Check sheet for the modelled part. Datum: model origin and axes. Units: mm. Face numbers are marked on the shaded views. Coordinates: 2 decimals unless noted, no trailing zeros. Loops run counter-clockwise (first coordinate to the right, second up) from the corner with the lowest first, then second, coordinate; pieces in that order, holes last. Notation, with made-up numbers: (1.25, -15) - (47.25, -15) arc R23 ccw to (47.25, -3) - close; hole circle Ø8 at (50, -14.5). An arc over 180 degrees is marked (long way). Use a Markdown table: item, result. Add a question column.
1) Thickness scan on line 1 (Z direction, x = -3, y = 9.5); line 2 (X direction, y = 9.5, z = -21.5); line 3 (Z direction, x = 2, y = 3.25). Record the ranges inside material, lowest first.
2) Go/stop test with flat-tipped pins: P1, Ø4.5, axis at x = 14, z = -68.5, coming from the +Y side; P2, Ø1.5, axis at y = 5, z = -24, coming from the +X side; P3, Ø1, axis at x = 10.5, y = 12, coming from the -Z side. Record where each tip stops, or that it passes through.
3) Draft check along Y on the marked faces 1, 2, 3 and 4. Enter one of: pulls with the +Y half, pulls with the -Y half, needs draft (parallel to the pull), parting line crosses it, or undercut.
4) Sectioned sample at B-B, the plane x = -0.75. Enter the section's corners in (y, z), then the cut area to 3 significant figures.
5) Sectioned sample at A-A, the plane y = 7.5. Enter the section's corners in (x, z).
6) Sectioned sample at C-C, the plane z = -52.5. Enter the section's corners in (x, y), then the cut area to 3 significant figures.
from build123d import *

# Parameters (mm, degrees)
SKETCH1_W           = 85.2
SKETCH1_H           = 18
SKETCH1_W_2         = 10
SKETCH1_H_2         = 12
BOSS_EXTRUDE1_DEPTH = 9
SKETCH2_W           = 5
SKETCH2_H           = 12
BOSS_EXTRUDE2_DEPTH = 6
FILLET1_R           = 2
FILLET2_R           = 1
FILLET3_R           = 4


with BuildPart() as part:
    # Sketch1 → Boss-Extrude1 (new, symmetric)
    with BuildSketch(Plane(origin=(0, 0, 0), x_dir=(0, 0, -1), z_dir=(1, 0, 0))):
        with Locations((42.6, 9)):
            Rectangle(SKETCH1_W, SKETCH1_H)
        with Locations((76.2, 9)):
            Rectangle(SKETCH1_W_2, SKETCH1_H_2, mode=Mode.SUBTRACT)
    extrude(amount=BOSS_EXTRUDE1_DEPTH, both=True)

    # Sketch2 → Boss-Extrude2 (add)
    with BuildSketch(Plane(origin=(9, 0, 0), x_dir=(0, 0, -1), z_dir=(1, 0, 0))):
        with Locations((68.7, 9)):
            Rectangle(SKETCH2_W, SKETCH2_H)
    extrude(amount=BOSS_EXTRUDE2_DEPTH)

    # Fillet1
    fillet1_edges = [part.edges().sort_by_distance(p)[0] for p in [
        (9, 15, -68.7),
        (9, 9, -66.2),
        (9, 3, -68.7),
    ]]
    fillet(fillet1_edges, radius=FILLET1_R)

    # Fillet2
    fillet2_edges = [part.edges().sort_by_distance(p)[0] for p in [
        (9, 9, -81.2),
        (9, 15, -76.2),
        (9, 3, -76.2),
    ]]
    fillet(fillet2_edges, radius=FILLET2_R)

    # Fillet3
    fillet3_edges = [part.edges().sort_by_distance(p)[0] for p in [
        (0, 18, -85.2),
        (0, 0, -85.2),
    ]]
    fillet(fillet3_edges, radius=FILLET3_R)


solid = part.part
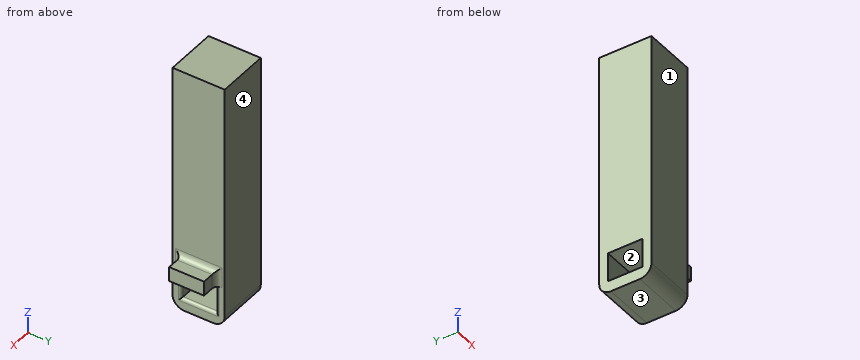
Solved:
| question | item | result |
|---|---|---|
| 1 | line 1 | z = -85.2 to -81.2, -71.2 to 0 |
| 1 | line 2 | x = -9 to 9 |
| 1 | line 3 | z = -85.13 to -81.2, -71.2 to 0 |
| 2 | P1 | stops at y = 15 |
| 2 | P2 | stops at x = 9 |
| 2 | P3 | stops at z = -71.2 |
| 3 | face 1 | pulls with the -Y half |
| 3 | face 2 | undercut |
| 3 | face 3 | needs draft |
| 3 | face 4 | pulls with the +Y half |
| 4 | outline | (0, -81.2) arc R4 ccw to (4, -85.2) - (14, -85.2) arc R4 ccw to (18, -81.2) - (18, 0) - (0, 0) - close; hole (3, -81.2) - (15, -81.2) - (15, -71.2) - (3, -71.2) - close |
| 4 | area | 1,410 mm2 |
| 5 | outline | (-9, -85.2) - (9, -85.2) - (9, -82.2) arc R1 ccw to (8, -81.2) - (-9, -81.2) - close; (-9, -71.2) - (15, -71.2) - (15, -66.2) - (11, -66.2) arc R2 cw to (9, -64.2) - (9, 0) - (-9, 0) - close |
| 6 | outline | (-9, 0) - (9, 0) - (9, 18) - (-9, 18) - close |
| 6 | area | 324 mm2 |
